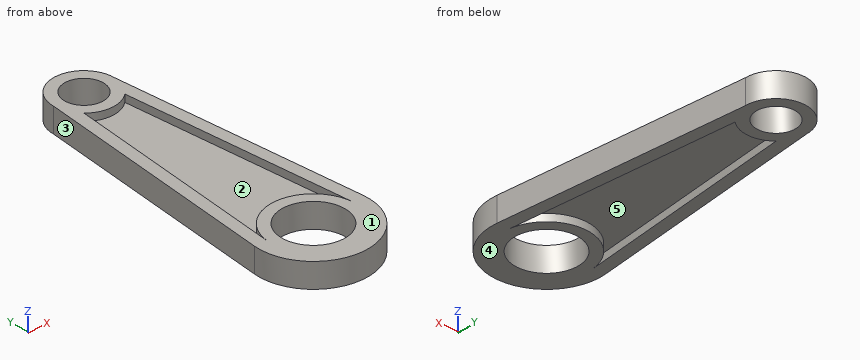
```python
from build123d import *

# Parameters (mm, degrees)
BOSS_EXTRUDE1_DEPTH = 10
CUT_EXTRUDE1_DEPTH  = 3
CUT_EXTRUDE2_START  = -3
CUT_EXTRUDE2_DEPTH  = 3
SKETCH8_R           = 17.5
SKETCH8_R_2         = 12.562549016
BOSS_EXTRUDE3_DEPTH = 10
SKETCH9_R           = 13
SKETCH9_R_2         = 8
CUT_EXTRUDE4_DEPTH  = 120.823194953


with BuildPart() as part:
    # Sketch2 → Boss-Extrude1 (new body)
    with BuildSketch(Plane.XY):
        with BuildLine():
            Line((-12.442858632, 105.897439267), (-22.397145538, 2.148923391))
            ThreePointArc((-22.397145538, 2.148923391), (0, -22.5), (22.397145538, 2.148923391))
            Line((22.397145538, 2.148923391), (12.442858632, 105.897439267))
            ThreePointArc((12.442858632, 105.897439267), (0, 117.203592938), (-12.442858632, 105.897439267))
        make_face()
    extrude(amount=BOSS_EXTRUDE1_DEPTH)

    # Sketch3 → Cut-Extrude1 (cut)
    with BuildSketch(Plane.XY.offset(10)):
        with BuildLine():
            Line((-7.465715179, 105.419900735), (-17.420002085, 1.67138486))
            ThreePointArc((-17.420002085, 1.67138486), (0, -17.5), (17.420002085, 1.67138486))
            Line((17.420002085, 1.67138486), (7.465715179, 105.419900735))
            ThreePointArc((7.465715179, 105.419900735), (0, 112.203592938), (-7.465715179, 105.419900735))
        make_face()
    extrude(amount=-CUT_EXTRUDE1_DEPTH, mode=Mode.SUBTRACT)

    # Sketch5 → Cut-Extrude2 (cut)
    with BuildSketch(Plane(origin=(0, 0, 0), x_dir=(-1, 0, 0), z_dir=(0, 0, -1)).offset(CUT_EXTRUDE2_START)):
        with BuildLine():
            Line((-7.465715179, 105.419900735), (-17.420002085, 1.67138486))
            ThreePointArc((-17.420002085, 1.67138486), (0, -17.5), (17.420002085, 1.67138486))
            Line((17.420002085, 1.67138486), (7.465715179, 105.419900735))
            ThreePointArc((7.465715179, 105.419900735), (0, 112.203592938), (-7.465715179, 105.419900735))
        make_face()
    extrude(amount=CUT_EXTRUDE2_DEPTH, mode=Mode.SUBTRACT)

    # Sketch8 → Boss-Extrude3 (add)
    with BuildSketch(Plane.XY):
        Circle(SKETCH8_R)
        with Locations((0, 104.703592938)):
            Circle(SKETCH8_R_2)
    extrude(amount=BOSS_EXTRUDE3_DEPTH)

    # Sketch9 → Cut-Extrude4 (cut, through all)
    with BuildSketch(Plane.XY.offset(10)):
        Circle(SKETCH9_R)
        with Locations((0, 104.703592938)):
            Circle(SKETCH9_R_2)
    extrude(amount=-CUT_EXTRUDE4_DEPTH, mode=Mode.SUBTRACT)


solid = part.part
```
The listing builds one solid part. Answer for the finished solid, in the listing's coordinates (mm). Face numbers are marked on the shaded views. A direction names the side the tool comes from. Round coordinates to 2 decimals unless told otherwise and drop trailing zeros. Loops run counter-clockwise (first coordinate to the right, second up) from the corner with the lowest first, then second, coordinate; pieces in that order, holes last.
1) A cutting plane is placed at C-C on z = 1.5. Determine the outline of the cut face in (x, y), plus the area to 3 significant figures.
Outcome:
outline: (-22.4, 2.15) arc R22.5 ccw (long way) to (22.4, 2.15) - (12.56, 104.65) arc R12.56 ccw (long way) to (-12.56, 104.65) - close; hole (-17.42, 1.67) arc R17.5 cw to (17.42, 1.67) - (8.43, 95.39) arc R12.56 cw to (-8.43, 95.39) - close; hole circle Ø26 at (0, 0); hole circle Ø16 at (0, 104.7)
area: 2,030 mm2
2) Given P1, Ø5, axis at x = 10, z = 3, coming from the -Y side; P2, Ø1, axis at y = 75.5, z = 6, coming from the -X side; P3, Ø6, axis at x = 14.5, y = 41, coming from the -Z side; P4, Ø1, axis at x = -10.5, y = 39, coming from the -Z side, each flat-ended and moving along its own axis, determine where each tip first touches the part or whether it passes through.
Outcome:
P1: stops at y = -21.21
P2: stops at x = -15.41
P3: stops at z = 0
P4: stops at z = 3
3) For the marked faces 4 and 5, determine the directions among +Z, -Z, +X, -X, +Y, -Y from which every point of the face is accessible in a straight line to the end or side of a thin tool.
Outcome:
face 4: -Z, +X, -X, +Y, -Y
face 5: -Z
4) A cutting plane is placed at A-A on y = 0. Determine the outline of the cut face in (x, z), plus the area to 3 significant figures.
Outcome:
outline: (-22.5, 0) - (-13, 0) - (-13, 10) - (-22.5, 10) - close; (13, 0) - (22.5, 0) - (22.5, 10) - (13, 10) - close
area: 190 mm2
5) For a pull along Y with two mould halves and no side action, classify the marked faces 1, 2 and 3 as released by +Y, released by -Y, zero draft, split by the parting line, or undercut.
Outcome:
face 1: zero draft
face 2: undercut
face 3: released by +Y
6) Consider line 1 (Y direction, x = 4.5, z = 1.25); line 2 (Z direction, x = 11, y = 58); line 3 (X direction, y = 90.5, z = 1.5). Determine where each line is inside the solid, lowest interval first.
Outcome:
line 1: y = -22.05 to -12.2, 12.2 to 16.91, 92.97 to 98.09, 111.32 to 116.43
line 2: z = 3 to 7
line 3: x = -13.92 to -8.9, 8.9 to 13.92
7) A cutting plane is placed at D-D on y = 25.5. Determine the outline of the cut face in (x, z).
Outcome:
outline: (-20.16, 0) - (-15.13, 0) - (-15.13, 3) - (15.13, 3) - (15.13, 0) - (20.16, 0) - (20.16, 10) - (15.13, 10) - (15.13, 7) - (-15.13, 7) - (-15.13, 10) - (-20.16, 10) - close
8) A cutting plane is placed at B-B on x = -3.5. Determine the outline of the cut face in (y, z).
Outcome:
outline: (-22.23, 0) - (-12.52, 0) - (-12.52, 10) - (-22.23, 10) - close; (12.52, 0) - (17.15, 0) - (17.15, 3) - (92.64, 3) - (92.64, 0) - (97.51, 0) - (97.51, 10) - (92.64, 10) - (92.64, 7) - (17.15, 7) - (17.15, 10) - (12.52, 10) - close; (111.9, 0) - (116.77, 0) - (116.77, 10) - (111.9, 10) - close
